The figure shows three views and two pictorial views of one solid part (mm, origin at its lowest corner). Answer the questions. A direction names the side the tool comes from. Give positions to 0.01 mm unless a question says otherwise; leave off trailing zeros. Loops run counter-clockwise (first coordinate to the right, second up) from the corner with the lowest first, then second, coordinate; pieces in that order, holes last. Notation, with made-up numbers: M 8.25,88.5 L 36.25,88.5 A12 ccw 36.25,107.5 Z; hole C 81.5,69.25 d5. An arc over 180 degrees is marked long. One line per item, written item: value. Start each with the question number.
Q1. A cutting plane is placed at D-D, the plane x = 1.5. Determine the outline of the cut face in (y, z).
Q2. A cutting plane is placed at C-C, the plane z = 0.8. Determine the outline of the cut face in (x, y).
Q3. Consider L1, parallel to Y at x = 8, z = 0.1; L2, parallel to X at y = 7.5, z = 0.25; L3, parallel to Y at x = 9, z = 0.7. Determine where each line is inside the solid, lowest interval first.
Q4. The mould has two halves that part along X. Classify the marked faces 1, 2 and 3: +X half, -X half, draft (parallel to the pull), parting line (faces both ways), or undercut.
Q5. A cutting plane is placed at A-A, the plane x = 8. Determine the outline of the cut face in (y, z).
Q6. A cutting plane is placed at B-B, the plane y = 8.75. Determine the outline of the cut face in (x, z).
Q7. For the marked faces 4 and 5, determine the directions among +Z, -Z, +X, -X, +Y, -Y from which every point of the face is accessible in a straight line to the end or side of a thin tool.
Q8. Flat-ended cylindrical pins translate along their axes: pin 1 (7 mm diameter, centred on x = 10.5, y = 6.5, fed in from -Z); pin 2 (1 mm diameter, centred on x = 14, y = 13.5, fed in from -Z). Find the tip coordinate at first contact, or state that the pin passes through.
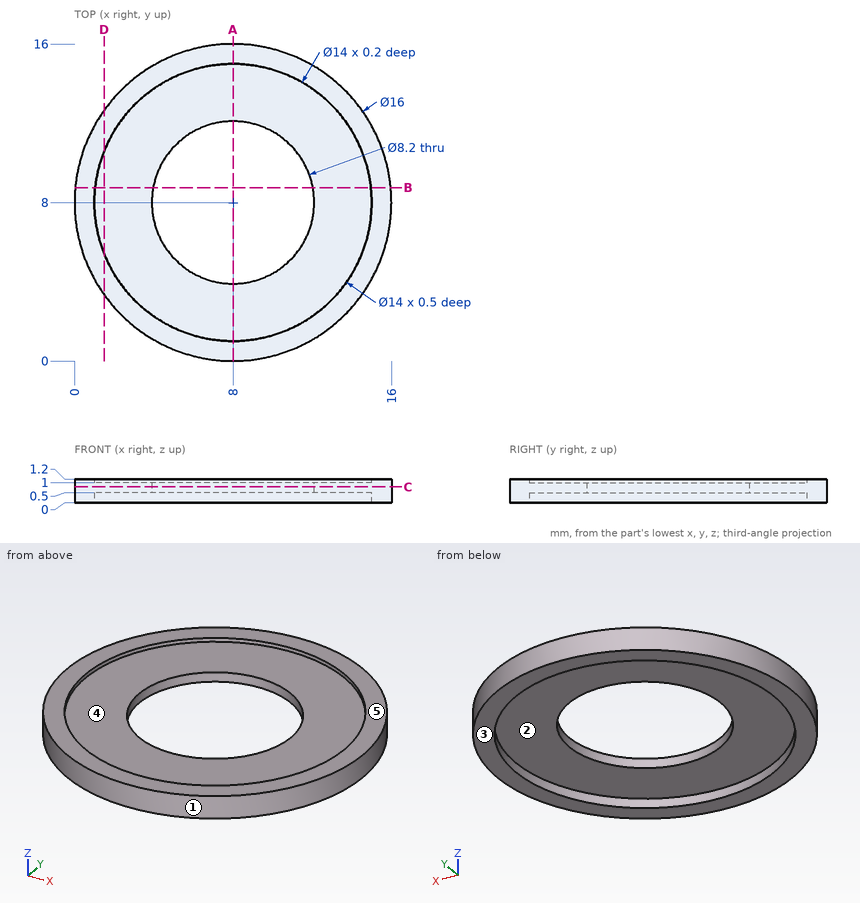
Answer block:
1. outline: M 3.34,0 L 5.4,0 L 5.4,0.5 L 10.6,0.5 L 10.6,0 L 12.66,0 L 12.66,1.2 L 10.6,1.2 L 10.6,1 L 5.4,1 L 5.4,1.2 L 3.34,1.2 Z
2. outline: C 8,8 d16; hole C 8,8 d8.2
3. L1: 0 to 1, 15 to 16
3. L2: 0.02 to 1.02, 14.98 to 15.98
3. L3: 0.06 to 4.02, 11.98 to 15.94
4. face 1: parting line
4. face 2: undercut
4. face 3: draft
5. outline: M 0,0 L 1,0 L 1,0.5 L 3.9,0.5 L 3.9,1 L 1,1 L 1,1.2 L 0,1.2 Z; M 12.1,0.5 L 15,0.5 L 15,0 L 16,0 L 16,1.2 L 15,1.2 L 15,1 L 12.1,1 Z
6. outline: M 0.04,0 L 1.04,0 L 1.04,0.5 L 3.97,0.5 L 3.97,1 L 1.04,1 L 1.04,1.2 L 0.04,1.2 Z; M 12.03,0.5 L 14.96,0.5 L 14.96,0 L 15.96,0 L 15.96,1.2 L 14.96,1.2 L 14.96,1 L 12.03,1 Z
7. face 4: +Z
7. face 5: +Z, +X, -X, +Y, -Y
8. pin 1: z = 0.5
8. pin 2: z = 0
